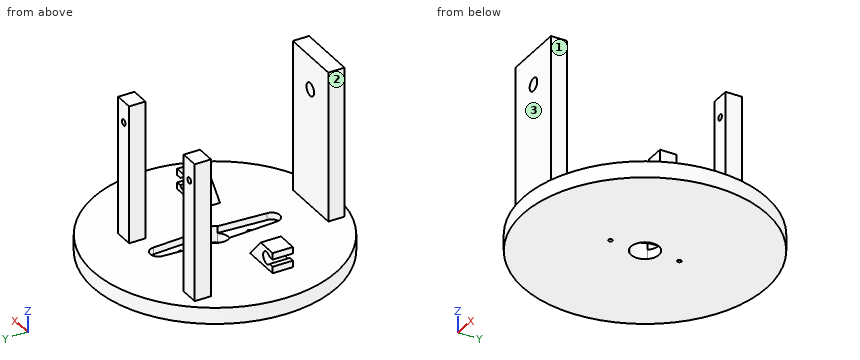
```python
from build123d import *
from build123d.topology import SkipClean

# Parameters (mm, degrees)
SKETCH1_R               = 30
BOSS_EXTRUDE1_DEPTH     = 4
CUT_EXTRUDE1_DEPTH      = 68.201190865
BOSS_EXTRUDE2_START     = -2.3
BOSS_EXTRUDE2_DEPTH     = 2.3
BOSS_EXTRUDE3_DEPTH     = 34
SKETCH5_R               = 0.75
CUT_EXTRUDE2_DEPTH      = 82.573644151
SKETCH6_R               = 0.500000007
SKETCH6_R_2             = 0.5
CUT_EXTRUDE3_DEPTH      = 10
SKETCH7_W               = 15
SKETCH7_H               = 4
BOSS_EXTRUDE4_DEPTH     = 37
SKETCH8_R               = 1.6
CUT_EXTRUDE4_DEPTH      = 37
SKETCH9_W               = 5.021529313
SKETCH9_H               = 4.978377583
SKETCH9_H_2             = 4.978377584
BOSS_EXTRUDE5_DEPTH     = 5
CUT_EXTRUDE5_DEPTH      = 5
CUT_EXTRUDE5_DEPTH_BACK = 15
BOSS_EXTRUDE6_DEPTH     = 4.978377584
BOSS_EXTRUDE7_DEPTH     = 4.978377584


with BuildPart() as part:
    # Sketch1 → Boss-Extrude1 (new body)
    with BuildSketch(Plane.XY):
        with Locations((-30.000000447, 0)):
            Circle(SKETCH1_R)
    extrude(amount=-BOSS_EXTRUDE1_DEPTH)

    # Sketch2 → Cut-Extrude1 (cut, through all)
    with BuildSketch(Plane.XY):
        with BuildLine():
            Line((-32.000000447, 13.925), (-32.700000447, 2.147673159))
            ThreePointArc((-32.700000447, 2.147673159), (-33.450000447, 0), (-32.700000447, -2.147673159))
            Line((-32.700000447, -2.147673159), (-32.000000447, -13.925))
            ThreePointArc((-32.000000447, -13.925), (-30.000000447, -15.925), (-28.000000447, -13.925))
            Line((-28.000000447, -13.925), (-27.300000447, -2.147673159))
            ThreePointArc((-27.300000447, -2.147673159), (-26.550000447, 0), (-27.300000447, 2.147673159))
            Line((-27.300000447, 2.147673159), (-28.000000447, 13.925))
            ThreePointArc((-28.000000447, 13.925), (-30.000000447, 15.925), (-32.000000447, 13.925))
        make_face()
    extrude(amount=-CUT_EXTRUDE1_DEPTH, mode=Mode.SUBTRACT)

    # Sketch3 → Boss-Extrude2 (add)
    with SkipClean():  # the faces are left unmerged after this step: merging them gives an invalid solid
        with BuildSketch(Plane(origin=(0, 0, -4), x_dir=(-1, 0, 0), z_dir=(0, 0, -1)).offset(BOSS_EXTRUDE2_START)):
            with BuildLine():
                Line((27.300000447, -2.147673159), (28.000000447, -13.925))
                ThreePointArc((28.000000447, -13.925), (30.000000447, -15.925), (32.000000447, -13.925))
                Line((32.000000447, -13.925), (32.700000447, -2.147673159))
                ThreePointArc((32.700000447, -2.147673159), (30.000000447, -3.45), (27.300000447, -2.147673159))
            make_face()
            with BuildLine():
                Line((32.000000447, 13.925), (32.700000447, 2.147673159))
                ThreePointArc((32.700000447, 2.147673159), (30.000000447, 3.45), (27.300000447, 2.147673159))
                Line((27.300000447, 2.147673159), (28.000000447, 13.925))
                ThreePointArc((28.000000447, 13.925), (30.000000447, 15.925), (32.000000447, 13.925))
            make_face()
        extrude(amount=BOSS_EXTRUDE2_DEPTH)

    # Sketch4 → Boss-Extrude3 (add)
    with SkipClean():  # the faces are left unmerged after this step: merging them gives an invalid solid
        with BuildSketch(Plane.XY):
            Polygon((-23.904804701, 13.547119626), (-19.304847529, 13.566969421), (-19.32210822, 17.566932179), (-23.922065393, 17.547082384), align=None)
            Polygon((-51.364549038, 13.42862498), (-46.764591865, 13.448474775), (-46.781852557, 17.448437533), (-51.381809729, 17.428587738), align=None)
        extrude(amount=BOSS_EXTRUDE3_DEPTH)

    # Sketch5 → Cut-Extrude2 (cut, through all)
    with SkipClean():  # the faces are left unmerged after this step: merging them gives an invalid solid
        with BuildSketch(Plane(origin=(-0.058902743, 13.650019772, 0), x_dir=(0.999990689598316, 0.004315172845242606, 0), z_dir=(0.004315172845242606, -0.9999906895983162, 0))):
            with Locations((-49.026123975, 28.818298908)):
                Circle(SKETCH5_R)
            with Locations((-21.526123975, 28.818298908)):
                Circle(SKETCH5_R)
        extrude(amount=-CUT_EXTRUDE2_DEPTH, mode=Mode.SUBTRACT)

    # Sketch6 → Cut-Extrude3 (cut)
    with SkipClean():  # the faces are left unmerged after this step: merging them gives an invalid solid
        with BuildSketch(Plane.XY):
            with Locations((-30.004011834, -8.464999042)):
                Circle(SKETCH6_R)
            with Locations((-29.99598906, 8.464999042)):
                Circle(SKETCH6_R_2)
        extrude(amount=-CUT_EXTRUDE3_DEPTH, mode=Mode.SUBTRACT)

    # Sketch7 → Boss-Extrude4 (add)
    with SkipClean():  # the faces are left unmerged after this step: merging them gives an invalid solid
        with BuildSketch(Plane.XY):
            with Locations((-30.000000447, -25.474087185)):
                Rectangle(SKETCH7_W, SKETCH7_H)
        extrude(amount=BOSS_EXTRUDE4_DEPTH)

    # Sketch8 → Cut-Extrude4 (cut)
    with SkipClean():  # the faces are left unmerged after this step: merging them gives an invalid solid
        with BuildSketch(Plane.XZ.offset(27.474087185)):
            with Locations((-29.878857802, 28.818298907)):
                Circle(SKETCH8_R)
        extrude(amount=-CUT_EXTRUDE4_DEPTH, mode=Mode.SUBTRACT)

    # Sketch9 → Boss-Extrude5 (add)
    with SkipClean():  # the faces are left unmerged after this step: merging them gives an invalid solid
        with BuildSketch(Plane.XY):
            with Locations((-12.324865315, -4.953083179)):
                Rectangle(SKETCH9_W, SKETCH9_H)
            with Locations((-47.324539451, -5.104114228)):
                Rectangle(SKETCH9_W, SKETCH9_H_2)
        extrude(amount=BOSS_EXTRUDE5_DEPTH)

    # Sketch11 → Cut-Extrude5 (cut, two sides: drawn at the far end of the back side and taken through both)
    with SkipClean():  # the faces are left unmerged after this step: merging them gives an invalid solid
        with BuildSketch(Plane.XZ.offset(7.44227197).offset(-CUT_EXTRUDE5_DEPTH_BACK)):
            with BuildLine():
                Line((-9.814100658, 1.616316037), (-11.112799865, 1.616316037))
                ThreePointArc((-11.112799865, 1.616316037), (-13.824865315, 2.5), (-11.112799865, 3.383683963))
                Line((-11.112799865, 3.383683963), (-9.814100658, 3.383683963))
                Line((-9.814100658, 3.383683963), (-9.814100658, 1.616316037))
            make_face()
            with BuildLine():
                Line((-49.835304107, 3.383683963), (-48.5366049, 3.383683963))
                ThreePointArc((-48.5366049, 3.383683963), (-45.82453945, 2.5), (-48.5366049, 1.616316037))
                Line((-48.5366049, 1.616316037), (-49.835304107, 1.616316037))
                Line((-49.835304107, 1.616316037), (-49.835304107, 3.383683963))
            make_face()
        extrude(amount=CUT_EXTRUDE5_DEPTH + CUT_EXTRUDE5_DEPTH_BACK, mode=Mode.SUBTRACT)

    # Sketch12 → Boss-Extrude6 (add)
    with SkipClean():  # the faces are left unmerged after this step: merging them gives an invalid solid
        with BuildSketch(Plane(origin=(0, -2.463894387, 0), x_dir=(1, 0, 0), z_dir=(0, 1, 0))):
            Polygon((-14.835629971, -5), (-19.32210822, 0), (-14.835629971, 0), align=None)
        extrude(amount=-BOSS_EXTRUDE6_DEPTH)

    # Sketch13 → Boss-Extrude7 (add)
    with SkipClean():  # the faces are left unmerged after this step: merging them gives an invalid solid
        with BuildSketch(Plane(origin=(0, -2.614925436, 0), x_dir=(1, 0, 0), z_dir=(0, 1, 0))):
            Polygon((-44.813774794, -5), (-44.813774794, 0), (-40.313774794, 0), align=None)
        extrude(amount=-BOSS_EXTRUDE7_DEPTH)


solid = part.part
```
Design review of the part built by this model. Coordinates are the model's own, in mm. Face numbers are marked on the shaded views. A direction names the side the tool comes from. Round coordinates to 2 decimals unless told otherwise and drop trailing zeros. Write each loop counter-clockwise with the first axis right and the second up, starting at its lowest first coordinate (ties: lowest second). Pieces come first, ordered by that corner, then holes.
Item 1: For the marked faces 1, 2 and 3, list the 3-axis set-ups (+Z, -Z, +X, -X, +Y, -Y) from which the entire face can be reached by the end or side of a thin tool; tool diameter is ignored.
Item 2: Clearance check with flat-ended pins moving along their axes: pin 1 Ø2.5 at (x, y) = (-12, -5.5) entering from +Z; pin 2 Ø3 at (x, y) = (-9.5, -14) entering from +Z; pin 3 Ø3 at (y, z) = (-25, 14) entering from +X. State where each tip first meets the part, or that it passes through.
Item 3: We need section D-D on x = -4.5. Write out the cut boundary in (y, z).
Item 4: We need section A-A on z = 21. Write out the cut boundary in (x, y).
Item 5: We need section C-C on z = 2.5. Write out the cut boundary in (x, y), and give its area (3 significant figures).
Item 6: We need section B-B on y = 0. Write out the cut boundary in (x, z).
Item 7: For probe 1 along X at (y, z) = (16.5, 5); probe 2 along Z at (x, y) = (-29, -8); probe 3 along Y at (x, z) = (-27.5, 23.5), list the stretches that pass through material, from the lowest coordinate up.
Returned:
1. face 1: +Z, +X, -Y
1. face 2: +Z, -X, +Y, -Y
1. face 3: +Z, +X, -X, -Y
2. pin 1: stops at z = 5
2. pin 2: stops at z = 0
2. pin 3: stops at x = -22.5
3. outline: (-15.8, -4) - (15.8, -4) - (15.8, 0) - (-15.8, 0) - close
4. outline: (-51.38, 17.43) - (-51.36, 13.43) - (-46.76, 13.45) - (-46.78, 17.45) - close; (-37.5, -27.47) - (-22.5, -27.47) - (-22.5, -23.47) - (-37.5, -23.47) - close; (-23.92, 17.55) - (-23.9, 13.55) - (-19.3, 13.57) - (-19.32, 17.57) - close
5. outline: (-51.38, 17.43) - (-51.36, 13.43) - (-46.76, 13.45) - (-46.78, 17.45) - close; (-45.82, -7.59) - (-42.56, -7.59) - (-42.56, -2.61) - (-45.82, -2.61) - close; (-37.5, -27.47) - (-22.5, -27.47) - (-22.5, -23.47) - (-37.5, -23.47) - close; (-23.92, 17.55) - (-23.9, 13.55) - (-19.3, 13.57) - (-19.32, 17.57) - close; (-17.08, -7.44) - (-13.82, -7.44) - (-13.82, -2.46) - (-17.08, -2.46) - close
5. area: 129 mm2
6. outline: (-60, -4) - (-33.45, -4) - (-33.45, 0) - (-60, 0) - close; (-26.55, -4) - (0, -4) - (0, 0) - (-26.55, 0) - close
7. probe 1: x = -51.38 to -46.78, -23.92 to -19.32
7. probe 2: z = -4 to -1.7
7. probe 3: y = -27.47 to -23.47
